Can you work these out from the model? Positions are in its coordinate system, mm. A direction names the side the tool comes from. Give positions to 0.01 mm unless a question says otherwise; leave off trailing zeros. Loops run counter-clockwise (first coordinate to the right, second up) from the corner with the lowest first, then second, coordinate; pieces in that order, holes last. Notation, with made-up numbers: M -34.75,9.25 L -2.75,9.25 A27 ccw -2.75,37.25 Z; hole C 25,19.25 d6. An arc over 180 degrees is marked long. Use CSV: the item, a comma, the result in double quotes.
from build123d import *

# Parameters (mm, degrees)
CYLINDER051_R     = 5.2
CYLINDER051_DEPTH = 6
CYLINDER052_R     = 3.3
CYLINDER052_DEPTH = 20
CYLINDER053_R     = 3.3
CYLINDER053_DEPTH = 20
CYLINDER050_R     = 5.2
CYLINDER050_DEPTH = 6
CYLINDER049_R     = 8.1
CYLINDER049_DEPTH = 20
CYLINDER048_R     = 8.1
CYLINDER048_DEPTH = 20
BOX002_W          = 200
BOX002_H          = 10
BOX002_DEPTH      = 25
FILLET_R          = 2


with BuildPart() as zylinder051:
    # Cylinder051 → Cylinder051 (new body)
    with BuildSketch(Plane(origin=(250, -22, 40), x_dir=(1, 0, 0), z_dir=(0, -1, 0))):
        Circle(CYLINDER051_R)
    extrude(amount=CYLINDER051_DEPTH)


with BuildPart() as zylinder052:
    # Cylinder052 → Cylinder052 (new body)
    with BuildSketch(Plane(origin=(80, -10, 40), x_dir=(1, 0, 0), z_dir=(0, -1, 0))):
        Circle(CYLINDER052_R)
    extrude(amount=CYLINDER052_DEPTH)


with BuildPart() as zylinder053:
    # Cylinder053 → Cylinder053 (new body)
    with BuildSketch(Plane(origin=(250, -10, 40), x_dir=(1, 0, 0), z_dir=(0, -1, 0))):
        Circle(CYLINDER053_R)
    extrude(amount=CYLINDER053_DEPTH)


with BuildPart() as fusion009:
    # Cylinder050 → Cylinder050 (new body)
    with BuildSketch(Plane(origin=(80, -22, 40), x_dir=(1, 0, 0), z_dir=(0, -1, 0))):
        Circle(CYLINDER050_R)
    extrude(amount=CYLINDER050_DEPTH)

    # Fusion009: union Zylinder051, Zylinder052, Zylinder053
    add(zylinder051.part)
    add(zylinder052.part)
    add(zylinder053.part)


with BuildPart() as zylinder049:
    # Cylinder049 → Cylinder049 (new body)
    with BuildSketch(Plane(origin=(250, 0, 40), x_dir=(1, 0, 0), z_dir=(0, -1, 0))):
        Circle(CYLINDER049_R)
    extrude(amount=CYLINDER049_DEPTH)


with BuildPart() as zylinder048:
    # Cylinder048 → Cylinder048 (new body)
    with BuildSketch(Plane(origin=(80, 0, 40), x_dir=(1, 0, 0), z_dir=(0, -1, 0))):
        Circle(CYLINDER048_R)
    extrude(amount=CYLINDER048_DEPTH)


with BuildPart() as obj1:
    # Box002 → Box002 (new body)
    with BuildSketch(Plane(origin=(66, -28, 27.5), x_dir=(1, 0, 0), z_dir=(0, 0, 1))):
        with Locations((100, 5)):
            Rectangle(BOX002_W, BOX002_H)
    extrude(amount=BOX002_DEPTH)

    # Cut008: cut Zylinder048
    add(zylinder048.part, mode=Mode.SUBTRACT)

    # Cut009: cut Zylinder049
    add(zylinder049.part, mode=Mode.SUBTRACT)

    # Cut010: cut Fusion009
    add(fusion009.part, mode=Mode.SUBTRACT)

    # Fillet
    fillet_edges = [obj1.edges().sort_by_distance(p)[0] for p in [
        (66, -28, 40),
        (66, -23, 52.5),
        (66, -18, 40),
        (66, -23, 27.5),
        (166, -28, 27.5),
        (266, -28, 40),
        (166, -28, 52.5),
        (166, -18, 52.5),
        (266, -23, 52.5),
        (166, -18, 27.5),
        (266, -18, 40),
        (266, -23, 27.5),
    ]]
    fillet(fillet_edges, radius=FILLET_R)


with BuildPart() as obj1_1:
    # Fillet placement: moved
    add(obj1.part.moved(Location((0, -5, 0))))


solid = obj1_1.part
Q1. If we mould it in two halves opening along X, with no side actions, what happens to faces 4 (the flat face through (165, -28, 27.5)), 5 (the flat face through (266, -28, 40)), 6 (the cylindrical face through (76.7, -26, 40.1))? For each: released by +X, released by -X, zero draft, split by the parting line, or undercut.
Model answer:
face 4,"zero draft"
face 5,"released by +X"
face 6,"undercut"
Q2. Please list where these lines run through material, in increasing order: L1, parallel to X at y = -24.6, z = 40; L2, parallel to X at y = -26.3, z = 40; L3, parallel to Z at x = 250, y = -28.25. Write a range as from..to.
Model answer:
L1,"66.04..71.9, 88.1..241.9, 258.1..265.96"
L2,"66..76.7, 83.3..246.7, 253.3..266"
L3,"27.5..34.8, 45.2..52.5"
Q3. For faces 1 (the cylindrical face through (76.167, -29.958, 43.514)), 2 (the flat face through (66, -28, 40)), 3 (the flat face through (249.9, -25, 36.5)), which set-ups out of +Z, -Z, +X, -X, +Y, -Y let a thin tool reach every point of the face, with its end or its side?
Model answer:
face 1,"-Y"
face 2,"+Z, -Z, -X, +Y, -Y"
face 3,"+Y"
Q4. I'm going to push flat-ended pins straight in: P1, Ø1, axis at x = 228, y = -24, coming from the +Z side; P2, Ø13, axis at x = 80, z = 40, coming from the +Y side. Where does each tip first touch, or does it pass through?
Model answer:
P1,"z = 52.44"
P2,"y = -25"
Q5. I want a section at A-A, the plane z = 40. State how many separate pieces and enclosed holes the cut face has, then the cut area to 3 significant figures.
Model answer:
separate pieces,"3"
enclosed holes,"0"
area,"1,780 mm2"
Q6. I want a section at B-B, the plane x = 80. Please give me the cut outline in (y, z), then the cut area to 3 significant figures.
Model answer:
outline,"M -33,29.5 A2 ccw -31,27.5 L -25,27.5 A2 ccw -23,29.5 L -23,31.9 L -25,31.9 L -25,36.7 L -27,36.7 L -27,34.8 L -33,34.8 Z; M -33,45.2 L -27,45.2 L -27,43.3 L -25,43.3 L -25,48.1 L -23,48.1 L -23,50.5 A2 ccw -25,52.5 L -31,52.5 A2 ccw -33,50.5 Z"
area,"139 mm2"
